from build123d import *

# Parameters (mm, degrees)
CROQUIS1_R              = 8.25
SALIENTE_EXTRUIR1_DEPTH = 36
CORTAR_EXTRUIR5_DEPTH   = 18
CORTAR_EXTRUIR7_DEPTH   = 15
CROQUIS23_R             = 7.75
SALIENTE_EXTRUIR4_DEPTH = 2
CROQUIS25_W             = 4
CROQUIS25_H             = 14
CORTAR_EXTRUIR8_DEPTH   = 15


with BuildPart() as part:
    # Croquis1 → Saliente-Extruir1 (new body)
    with BuildSketch(Plane(origin=(0, 0, 0), x_dir=(1, 0, 0), z_dir=(0, 1, 0))):
        Circle(CROQUIS1_R)
    extrude(amount=SALIENTE_EXTRUIR1_DEPTH)

    # Croquis3 → Cortar-Extruir5 (cut, symmetric)
    with BuildSketch(Plane(origin=(0, 0, 0), x_dir=(0, 0, -1), z_dir=(1, 0, 0))):
        Polygon((8.25, 0), (8.25, 14), (3.5, 4), (3.5, 0), align=None)
    extrude(amount=CORTAR_EXTRUIR5_DEPTH, both=True, mode=Mode.SUBTRACT)

    # Croquis18 → Revolución1 (revolve)
    with BuildSketch(Plane(origin=(0, 0, 0), x_dir=(0, 0, -1), z_dir=(1, 0, 0))):
        with BuildLine():
            Line((0, 8.25), (0, -8.25))
            ThreePointArc((0, -8.25), (8.25, 0), (0, 8.25))
        make_face()
    revolve(axis=Axis((0, 8.25, 0), (0, -1, 0)))

    # Croquis20 → Cortar-Revolución1 (revolve, cut)
    with BuildSketch(Plane(origin=(0, 36, 0), x_dir=(1, 0, 0), z_dir=(0, 1, 0))):
        with BuildLine():
            Line((-8, 0), (8, 0))
            ThreePointArc((8, 0), (0, 8), (-8, 0))
        make_face()
    revolve(axis=Axis((-8, 36, 0), (1, 0, 0)), mode=Mode.SUBTRACT)

    # Croquis24 → Cortar-Extruir7 (cut, symmetric)
    with BuildSketch(Plane(origin=(0, 0, 0), x_dir=(0, 0, -1), z_dir=(1, 0, 0))):
        with BuildLine():
            Line((-5.973353696, 36), (8.25, 36))
            Line((8.25, 36), (8.25, 34.163037065))
            add(Edge.make_bspline(
                [(-5.973353696, 36), (-1.37807863, 34.604512728), (3.281869782, 34.274988011), (8.25, 34.163037065)],
                knots=[0, 0, 0, 0, 1, 1, 1, 1], degree=3))
        make_face()
    extrude(amount=CORTAR_EXTRUIR7_DEPTH, both=True, mode=Mode.SUBTRACT)

    # Croquis23 → Saliente-Extruir4 (add, symmetric)
    with BuildSketch(Plane(origin=(0, 0, 0), x_dir=(0, 0, -1), z_dir=(1, 0, 0))):
        with Locations((0, 36)):
            Circle(CROQUIS23_R)
    extrude(amount=SALIENTE_EXTRUIR4_DEPTH, both=True)

    # Croquis25 → Cortar-Extruir8 (cut, symmetric)
    with BuildSketch(Plane.XY):
        with Locations((0, -1.25)):
            Rectangle(CROQUIS25_W, CROQUIS25_H)
    extrude(amount=CORTAR_EXTRUIR8_DEPTH, both=True, mode=Mode.SUBTRACT)


solid = part.part
Input: part model. Units: mm. Frame: model coordinates. A direction names the side the tool comes from. Give positions to 0.01 mm unless a question says otherwise; leave off trailing zeros. Write each loop counter-clockwise with the first axis right and the second up, starting at its lowest first coordinate (ties: lowest second). Pieces come first, ordered by that corner, then holes. Notation, with made-up numbers: (44, 35.5) -> (97, 35.5) arc R25 ccw to (97, 50.5) -> close; hole circle Ø7 at (30.25, -16). An arc over 180 degrees is marked (long way). Use one line per item in the form item = value. Start each with the question number.
1) Section query A-A on y = 1.5. Return the cut outline in (x, z).
2) Draft query along Y for faces 1 (the flat face through (-2, -1, 0)), 2 (the flat face through (0.1, 9.07, -5.91)), 3 (the flat face through (0, 5.75, 1)). Return one class per face: pulls with the +Y half, pulls with the -Y half, needs draft (parallel to the pull), parting line crosses it, or undercut.
3) Ray query, probe 1 along X at (y, z) = (32, 3.5); probe 2 along Y at (x, z) = (1.25, -5); probe 3 along X at (y, z) = (31, -3.75). Return the intervals inside material, ascending. Write a range as from..to.
4) Section query C-C on y = 26.5. Return the cut outline in (x, z).
5) Set-up query: faces 4 (the cylindrical face through (0.028, 43.684, 1.009)), 5 (the flat face through (2, 36, 0)), 6 (the flat face through (2, -1, 0)), 7 (the flat face through (7.1, 3, -3.5)), 8 (the flat face through (-7.1, 3, -3.5)). Return all of +Z, -Z, +X, -X, +Y, -Y with unobstructed straight access to the full face (end or side cutting, diameter ignored); none if empty.
6) Pin query (flat end, axial travel): pin 1 (8 mm diameter, centred on x = -4, y = 9.5, fed in from -Z); pin 2 (4 mm diameter, centred on x = -0.5, y = 4.5, fed in from -Z); pin 3 (0.9 mm diameter, centred on x = 7, y = 3, fed in from -Z). Return the tip coordinate at first contact, or that it passes through.
7) Section query D-D on y = 10. Return the cut outline in (x, z).
8) Section query B-B on z = 7. Return the cut outline in (x, y).
Outcome:
q1.outline = (-7.47, -3.5) -> (-7.32, -3.5) arc R8.11 ccw to (-2, -7.86) -> (-2, 8) arc R8.25 ccw to start; (2, -7.86) arc R8.11 ccw to (7.32, -3.5) -> (7.47, -3.5) arc R8.25 ccw to (2, 8) -> close
q2.face_1 = needs draft
q2.face_2 = undercut
q2.face_3 = pulls with the -Y half
q3.probe_1 = -7.47..-5.98, -2..2, 5.98..7.47
q3.probe_2 = 5.75..6.44, 7.16..29.88, 30.08..41.92
q3.probe_3 = -7.35..-4.99, -2..2, 4.99..7.35
q4.outline = circle Ø16.5 at (0, 0)
q5.face_4 = none
q5.face_5 = +Y
q5.face_6 = +Z, -Z, -Y
q5.face_7 = -Z, +X
q5.face_8 = -Z, -X
q6.pin_1 = -7.87
q6.pin_2 = -7.35
q6.pin_3 = -4.09
q7.outline = (-5.27, -6.35) -> (5.27, -6.35) arc R8.25 ccw (long way) to start
q8.outline = (-4.37, 0) arc R4.37 ccw to (-2, -3.88) -> (-2, 5.75) -> (2, 5.75) -> (2, -3.88) arc R4.37 ccw to (4.37, 0) -> (4.37, 36) -> (3.87, 36) arc R3.87 cw to (2, 32.68) -> (2, 39.33) -> (-2, 39.33) -> (-2, 32.68) arc R3.87 cw to (-3.87, 36) -> (-4.37, 36) -> close; hole (-1.98, 32.67) arc R3.87 ccw to (1.98, 32.67) -> close
